CAD build for the part. Positions are in the model's coordinates, mm. Give positions to 0.01 mm unless a question says otherwise; leave off trailing zeros. Order: outer loops, then holes, each group sorted by start corner. A loop starts at its lowest first (then second) coordinate and runs counter-clockwise, first axis right, second up. Notation, with made-up numbers: (-9, -1.75) -> (11, -1.75) arc R11 ccw to (11, 9.25) -> close; hole circle Ø10 at (-7.75, -39.5). An arc over 180 degrees is marked (long way). Use one line per item in the form item = value. Start each with the question number.
1) Cut at A-A, the plane y = 685. Give the cut face in (x, z), and give its area (3 significant figures).
2) Cut at C-C, the plane z = 0. State how many separate pieces and enclosed holes the cut face has, and give its area (3 significant figures).
3) Drop a flat-ended pin along its axis: P1, Ø5, axis at y = 445, z = -0.5, coming from the -X side. Give the stop position or say it passes through.
4) Probe line 1 (X direction, y = 328, z = -9); line 2 (Z direction, x = -4.25, y = 535); line 3 (X direction, y = 462.5, z = -11). List the from-to ranges inside material, lowest first.
5) Cut at B-B, the plane y = 420. Give the cut face in (x, z), and give its area (3 significant figures).
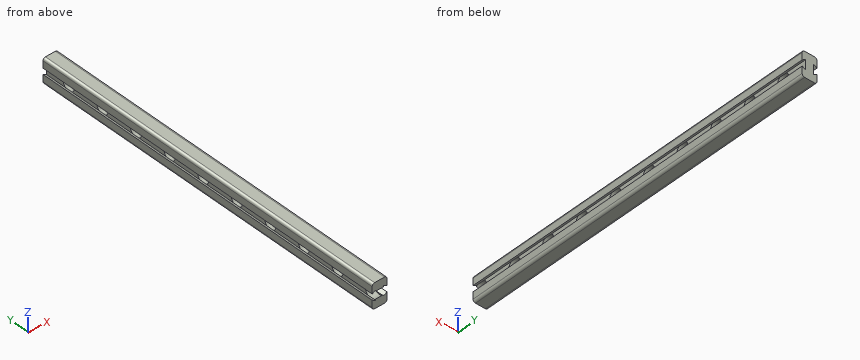
from build123d import *

# Parameters (mm, degrees)
BOSS_EXTRUDE1_DEPTH     = 735
SKETCH3_R               = 12.5
CUT_EXTRUDE2_DEPTH      = 8
CUT_EXTRUDE2_DEPTH_BACK = 8
FILLET1_R               = 5


with BuildPart() as part:
    # Sketch1 → Boss-Extrude1 (new body)
    with BuildSketch(Plane(origin=(0, 0, 0), x_dir=(1, 0, 0), z_dir=(0, 1, 0))):
        Polygon((15, 25), (15, 5.958548116), (8, 10), (8, -10), (15, -5.958548116), (15, -25), (-15, -25), (-15, -5.958548116), (-8, -10), (-8, 10), (-15, 5.958548116), (-15, 25), align=None)
    extrude(amount=BOSS_EXTRUDE1_DEPTH)

    # Sketch3 → Cut-Extrude2 (cut, two sides)
    with BuildSketch(Plane(origin=(0, 0, 0), x_dir=(0, 0, -1), z_dir=(1, 0, 0))) as cut_extrude2_sk:
        with Locations((0, 685)):
            Circle(SKETCH3_R)
        with Locations((0, 610)):
            Circle(SKETCH3_R)
        with Locations((0, 535)):
            Circle(SKETCH3_R)
        with Locations((0, 460)):
            Circle(SKETCH3_R)
        with Locations((0, 385)):
            Circle(SKETCH3_R)
        with Locations((0, 310)):
            Circle(SKETCH3_R)
        with Locations((0, 235)):
            Circle(SKETCH3_R)
        with Locations((0, 160)):
            Circle(SKETCH3_R)
        with Locations((0, 85)):
            Circle(SKETCH3_R)
        with Locations((0, 10)):
            Circle(SKETCH3_R)
        with Locations((0, -65)):
            Circle(SKETCH3_R)
    extrude(amount=CUT_EXTRUDE2_DEPTH, mode=Mode.SUBTRACT)
    extrude(cut_extrude2_sk.sketch, amount=-CUT_EXTRUDE2_DEPTH_BACK, mode=Mode.SUBTRACT)

    # Fillet1
    fillet1_edges = [part.edges().sort_by_distance(p)[0] for p in [
        (15, 367.5, -25),
        (15, 367.5, 25),
        (-15, 367.5, 25),
        (-15, 367.5, -25),
    ]]
    fillet(fillet1_edges, radius=FILLET1_R)


solid = part.part
Result:
q1.outline = (-15, -20) arc R5 ccw to (-10, -25) -> (10, -25) arc R5 ccw to (15, -20) -> (15, -5.96) -> (8, -10) -> (8, -12.5) -> (-8, -12.5) -> (-8, -10) -> (-15, -5.96) -> close; (-15, 5.96) -> (-8, 10) -> (-8, 12.5) -> (8, 12.5) -> (8, 10) -> (15, 5.96) -> (15, 20) arc R5 ccw to (10, 25) -> (-10, 25) arc R5 ccw to (-15, 20) -> close
q1.area = 855 mm²
q2.separate_pieces = 10
q2.enclosed_holes = 0
q2.area = 7,800 mm²
q3.P1 = -8
q4.line_1 = -15 to -9.73, -8 to 8, 9.73 to 15
q4.line_2 = -25 to -12.5, 12.5 to 25
q4.line_3 = -15 to -8, 8 to 15
q5.outline = (-15, -20) arc R5 ccw to (-10, -25) -> (10, -25) arc R5 ccw to (15, -20) -> (15, -5.96) -> (8, -10) -> (8, 10) -> (15, 5.96) -> (15, 20) arc R5 ccw to (10, 25) -> (-10, 25) arc R5 ccw to (-15, 20) -> (-15, 5.96) -> (-8, 10) -> (-8, -10) -> (-15, -5.96) -> close
q5.area = 1,260 mm²
